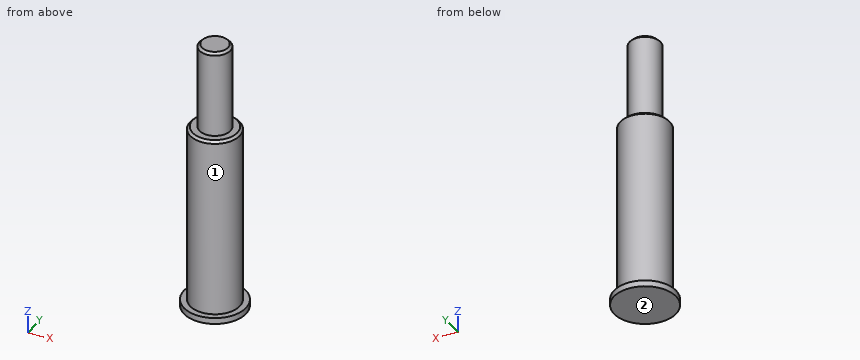
from build123d import *

# Parameters (mm, degrees)
SKETCH1_R           = 4
BOSS_EXTRUDE1_DEPTH = 29.3
SKETCH5_R           = 2.5
BOSS_EXTRUDE4_DEPTH = 14
SKETCH6_R           = 5
BOSS_EXTRUDE5_DEPTH = 1
CHAMFER1_SIZE       = 0.4


with BuildPart() as part:
    # Sketch1 → Boss-Extrude1 (new body)
    with BuildSketch(Plane.XY):
        Circle(SKETCH1_R)
    extrude(amount=BOSS_EXTRUDE1_DEPTH)

    # Sketch5 → Boss-Extrude4 (add)
    with BuildSketch(Plane.XY.offset(29.3)):
        Circle(SKETCH5_R)
    extrude(amount=BOSS_EXTRUDE4_DEPTH)

    # Sketch6 → Boss-Extrude5 (add)
    with BuildSketch(Plane(origin=(0, 0, 0), x_dir=(-1, 0, 0), z_dir=(0, 0, -1))):
        Circle(SKETCH6_R)
    extrude(amount=BOSS_EXTRUDE5_DEPTH)

    # Chamfer1
    chamfer1_edges = [part.edges().sort_by_distance(p)[0] for p in [
        (-4, 0, 29.3),
        (-2.5, 0, 43.3),
    ]]
    chamfer(chamfer1_edges, length=CHAMFER1_SIZE)


solid = part.part
CAD build for the part. Positions are in the model's coordinates, mm. Face numbers are marked on the shaded views. A direction names the side the tool comes from. Give positions to 0.01 mm unless a question says otherwise; leave off trailing zeros. Loops run counter-clockwise (first coordinate to the right, second up) from the corner with the lowest first, then second, coordinate; pieces in that order, holes last. Notation, with made-up numbers: M 10.25,-34 L 63.25,-34 A34 cw 63.25,5 Z; hole C -22.75,20.25 d2. An arc over 180 degrees is marked long. Answer in a Markdown table with one row per item. Add a question column.
Item 1: Drop flat-ended pins along their axis: P1, Ø5, axis at y = -1.5, z = 23.5, coming from the -X side; P2, Ø1, axis at y = 3.5, z = 22, coming from the -X side; P3, Ø2, axis at x = -3.5, z = 24.5, coming from the +Y side. Give the stop position or say it passes through.
Item 2: Probe probe 1 along Z at (x, y) = (3.25, -1.5); probe 2 along Z at (x, y) = (-1.5, 4); probe 3 along Y at (x, z) = (0.75, 26). List the from-to ranges inside material, lowest first.
Item 3: Band-saw the part on A-A on y = 0. Give the cut face in (x, z), then the cut area to 3 significant figures.
Item 4: Band-saw the part on D-D on z = 9. Give the cut face in (x, y).
Item 5: Band-saw the part on C-C on z = 39. Give the cut face in (x, y), then the cut area to 3 significant figures.
Item 6: Tool access for the marked faces 1 and 2: list every direction of +Z, -Z, +X, -X, +Y, -Y with a clear straight run to the whole face (end or side of a thin tool).
Reply:
| question | item | result |
|---|---|---|
| 1 | P1 | stops at x = -4 |
| 1 | P2 | stops at x = -2.65 |
| 1 | P3 | stops at y = 3.12 |
| 2 | probe 1 | z = -1 to 29.3 |
| 2 | probe 2 | z = -1 to 0 |
| 2 | probe 3 | y = -3.93 to 3.93 |
| 3 | outline | M -5,-1 L 5,-1 L 5,0 L 4,0 L 4,28.9 L 3.6,29.3 L 2.5,29.3 L 2.5,42.9 L 2.1,43.3 L -2.1,43.3 L -2.5,42.9 L -2.5,29.3 L -3.6,29.3 L -4,28.9 L -4,0 L -5,0 Z |
| 3 | area | 314 mm^2 |
| 4 | outline | C 0,0 d8 |
| 5 | outline | C 0,0 d5 |
| 5 | area | 19.6 mm^2 |
| 6 | face 1 | +Z |
| 6 | face 2 | -Z, +X, -X, +Y, -Y |
